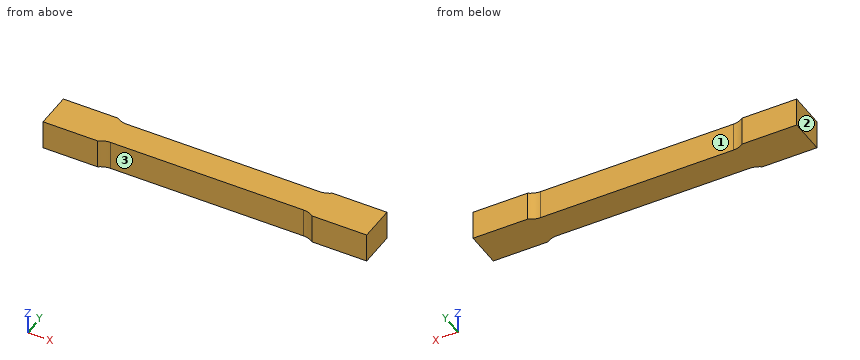
from build123d import *

# Parameters (mm, degrees)
F1_DEPTH = 20


with BuildPart() as f1:
    # F0 (on Top) → F1 (new body, symmetric)
    with BuildSketch(Plane.XY):
        with BuildLine():
            Line((132.5, 20), (0, 20))
            Line((0, 20), (-132.5, 20))
            ThreePointArc((-132.5, 20), (-140.405694, 21.282918), (-147.5, 25))
            Line((-147.5, 25), (-222.5, 25))
            Line((-222.5, 25), (-222.5, 0))
            Line((-222.5, 0), (-222.5, -25))
            Line((-222.5, -25), (-147.5, -25))
            ThreePointArc((-147.5, -25), (-140.405694, -21.282918), (-132.5, -20))
            Line((-132.5, -20), (0, -20))
            Line((0, -20), (132.5, -20))
            ThreePointArc((132.5, -20), (140.405694, -21.282918), (147.5, -25))
            Line((147.5, -25), (222.5, -25))
            Line((222.5, -25), (222.5, 0))
            Line((222.5, 0), (222.5, 25))
            Line((222.5, 25), (147.5, 25))
            ThreePointArc((147.5, 25), (140.405694, 21.282918), (132.5, 20))
        make_face()
    extrude(amount=F1_DEPTH, both=True)


solid = f1.part
For this review, take the finished solid that the model builds, in its own axes (mm). Face numbers are marked on the shaded views. A direction names the side the tool comes from. Give positions to 0.01 mm unless a question says otherwise; leave off trailing zeros. Order: outer loops, then holes, each group sorted by start corner. A loop starts at its lowest first (then second) coordinate and runs counter-clockwise, first axis right, second up. Notation, with made-up numbers: (56.5, 53) - (89.5, 53) arc R10 cw to (89.5, 65) - close; hole circle Ø2 at (51, 46). An arc over 180 degrees is marked (long way). Answer as a JSON object with one key per item and string values. Group by question number.
Item 1: Take a section at B-B on x = -100.5. Give the boundary of the cut face in (y, z), and give its area (3 significant figures).
Item 2: Clearance check with flat-ended pins moving along their axes: pin 1 Ø12 at (x, z) = (-144.5, 10) entering from +Y; pin 2 Ø3 at (x, z) = (139.5, -4.5) entering from +Y; pin 3 Ø5 at (x, z) = (24, 10) entering from +Y; pin 4 Ø12 at (x, z) = (-139, -10.5) entering from -Y. State where each tip first meets the part, or that it passes through.
Item 3: Take a section at A-A on z = -13.5. Give the boundary of the cut face in (x, y).
Item 4: Machinability: for the marked faces 1, 2 and 3, which of the approach directions +Z, -Z, +X, -X, +Y, -Y give a long, thin tool a straight path to every point of the face, cutting with its end or side? Answer none if there is none.
Item 5: Wall thickness on line 1 along Y through (x, z) = (-113, 11.5); line 2 along X through (y, z) = (-22.5, -8.5); line 3 along Y through (x, z) = (-142.5, 4.5): over which ranges is each line inside the solid? List them lowest first.
Reported:
{
 "1": {"outline": "(-20, -20) - (20, -20) - (20, 20) - (-20, 20) - close", "area": "1,600 mm^2"},
 "2": {"pin 1": "y = 25", "pin 2": "y = 21.49", "pin 3": "y = 20", "pin 4": "y = -23.35"},
 "3": {"outline": "(-222.5, -25) - (-147.5, -25) arc R25 cw to (-132.5, -20) - (132.5, -20) arc R25 cw to (147.5, -25) - (222.5, -25) - (222.5, 25) - (147.5, 25) arc R25 cw to (132.5, 20) - (-132.5, 20) arc R25 cw to (-147.5, 25) - (-222.5, 25) - close"},
 "4": {"face 1": "+Z, -Z, +Y", "face 2": "+Z, -Z, -X, +Y, -Y", "face 3": "+Z, -Z, -Y"},
 "5": {"line 1": "-20 to 20", "line 2": "-222.5 to -143.4, 143.4 to 222.5", "line 3": "-22.09 to 22.09"}
}
